Source: CAD feature listing. Evaluate the final solid. Frame: model axes, mm. A direction names the side the tool comes from. Give positions to 0.01 mm unless a question says otherwise; leave off trailing zeros. Write each loop counter-clockwise with the first axis right and the second up, starting at its lowest first coordinate (ties: lowest second). Pieces come first, ordered by that corner, then holes. Notation, with made-up numbers: (-37.5, 73.5) - (2.5, 73.5) arc R26 cw to (2.5, 95.5) - close; hole circle Ø7 at (33, -11.75). An arc over 180 degrees is marked (long way). One line per question, with ' | ' between items. Start each with the question number.
(1) Section A-A, the plane x = 77. Return loops of the section in (y, z).
(2) Section B-B, the plane z = 3.55. State how many separate pieces and enclosed holes the cut face has, plus the area to 3 significant figures.
(3) Draft query along Y for faces 3 (the flat face through (110, 52, 2)), 4 (the flat face through (-115, 36, 2)), 5 (the flat face through (-2, 0, 2)), 6 (the flat face through (107, 35, 2)). Return one class per face: +Y half, -Y half, draft (parallel to the pull), parting line (faces both ways), or undercut.
(4) Ray query, line 1 (X direction, y = 39, z = 1.15); line 2 (Y direction, x = 6, z = 2.95). Return the intervals inside material, ascending. Write a range as [from, to].
(5) Access query for faces 1 (the flat face through (110, 22, 2)), 2 (the flat face through (-2, 37, 0)). Directions: +Z, -Z, +X, -X, +Y, -Y. A direction counts if a zero-diameter tool reaches every point of the face in a straight line with its end or side. Return the directions, or none.
(6) Pin query (flat end, axial travel): pin 1 (2.5 mm diameter, centred on x = -107.5, y = 15, fed in from +Z). Return the tip coordinate at first contact, or that it passes through.
```python
from build123d import *

# Parameters (mm, degrees)
ESQUISSE1_W        = 230
ESQUISSE1_H        = 73
ESQUISSE1_R        = 1.5
ESQUISSE1_W_2      = 5
ESQUISSE1_H_2      = 5
BOSS_EXTRU_1_DEPTH = 5
CONG_1_R           = 5


with BuildPart() as part:
    # Esquisse1 → Boss.-Extru.1 (new body)
    with BuildSketch(Plane.XY):
        with Locations((0, 36.5)):
            Rectangle(ESQUISSE1_W, ESQUISSE1_H)
        with Locations((107.5, 45)):
            Circle(ESQUISSE1_R, mode=Mode.SUBTRACT)
        with Locations((107.5, 15)):
            Circle(ESQUISSE1_R, mode=Mode.SUBTRACT)
        with Locations(Location((-107.5, 15, 0), (0, 0, 180))):
            Circle(ESQUISSE1_R, mode=Mode.SUBTRACT)
        with Locations(Location((-107.5, 45, 0), (0, 0, 180))):
            Circle(ESQUISSE1_R, mode=Mode.SUBTRACT)
        with Locations(Location((0, 65.5, 0), (0, 0, 90))):
            Circle(ESQUISSE1_R, mode=Mode.SUBTRACT)
        with Locations(Location((70, 65.5, 0), (0, 0, 90))):
            Circle(ESQUISSE1_R, mode=Mode.SUBTRACT)
        with Locations((-70, 65.5)):
            Circle(ESQUISSE1_R, mode=Mode.SUBTRACT)
        with Locations((107.5, 37.5)):
            Rectangle(ESQUISSE1_W_2, ESQUISSE1_H_2, mode=Mode.SUBTRACT)
        with Locations((107.5, 52.5)):
            Rectangle(ESQUISSE1_W_2, ESQUISSE1_H_2, mode=Mode.SUBTRACT)
        with Locations((107.5, 7.5)):
            Rectangle(ESQUISSE1_W_2, ESQUISSE1_H_2, mode=Mode.SUBTRACT)
        with Locations((107.5, 22.5)):
            Rectangle(ESQUISSE1_W_2, ESQUISSE1_H_2, mode=Mode.SUBTRACT)
        with Locations((-107.5, 7.5)):
            Rectangle(ESQUISSE1_W_2, ESQUISSE1_H_2, mode=Mode.SUBTRACT)
        with Locations((-107.5, 22.5)):
            Rectangle(ESQUISSE1_W_2, ESQUISSE1_H_2, mode=Mode.SUBTRACT)
        with Locations((-107.5, 37.5)):
            Rectangle(ESQUISSE1_W_2, ESQUISSE1_H_2, mode=Mode.SUBTRACT)
        with Locations((-107.5, 52.5)):
            Rectangle(ESQUISSE1_W_2, ESQUISSE1_H_2, mode=Mode.SUBTRACT)
        with Locations((7.5, 65.5)):
            Rectangle(ESQUISSE1_W_2, ESQUISSE1_H_2, mode=Mode.SUBTRACT)
        with Locations((-7.5, 65.5)):
            Rectangle(ESQUISSE1_W_2, ESQUISSE1_H_2, mode=Mode.SUBTRACT)
        with Locations((77.5, 65.5)):
            Rectangle(ESQUISSE1_W_2, ESQUISSE1_H_2, mode=Mode.SUBTRACT)
        with Locations((62.5, 65.5)):
            Rectangle(ESQUISSE1_W_2, ESQUISSE1_H_2, mode=Mode.SUBTRACT)
        with Locations((-77.5, 65.5)):
            Rectangle(ESQUISSE1_W_2, ESQUISSE1_H_2, mode=Mode.SUBTRACT)
        with Locations((-62.5, 65.5)):
            Rectangle(ESQUISSE1_W_2, ESQUISSE1_H_2, mode=Mode.SUBTRACT)
    extrude(amount=BOSS_EXTRU_1_DEPTH)

    # Congé1
    cong_1_edges = [part.edges().sort_by_distance(p)[0] for p in [
        (-115, 73, 2.5),
        (115, 73, 2.5),
        (115, 0, 2.5),
        (-115, 0, 2.5),
    ]]
    fillet(cong_1_edges, radius=CONG_1_R)


solid = part.part
```
Check sheet entries:
1) outline: (0, 0) - (63, 0) - (63, 5) - (0, 5) - close; (68, 0) - (73, 0) - (73, 5) - (68, 5) - close
2) separate pieces: 1 | enclosed holes: 21 | area: 16,400 mm²
3) face 3: undercut | face 4: draft | face 5: -Y half | face 6: undercut
4) line 1: [-115, -110], [-105, 105], [110, 115] | line 2: [0, 63], [68, 73]
5) face 1: +Z, -Z | face 2: -Z, +X, -X, +Y, -Y
6) pin 1: through
